```python
from build123d import *

# Parameters (mm, degrees)
SKETCH1_W               = 38.1508
SKETCH1_H               = 9.525
CUT_EXTRUDE1_DEPTH      = 55.787705795
CUT_EXTRUDE1_DEPTH_BACK = 55.787705795
SKETCH2_R               = 11.8745
SKETCH2_R_2             = 3.175
CUT_EXTRUDE2_DEPTH      = 55.787705795
CUT_EXTRUDE2_DEPTH_BACK = 55.787705795
SKETCH3_R               = 3.175
SKETCH4_R               = 2.3749
CUT_EXTRUDE3_DEPTH      = 6.35
CIRPATTERN1_COUNT       = 3


with BuildPart() as part:
    # Sketch1 → Revolve1 (revolve)
    with BuildSketch(Plane.XY, mode=Mode.PRIVATE) as revolve1_sk:
        with Locations((19.0754, 4.7625)):
            Rectangle(SKETCH1_W, SKETCH1_H)
    revolve(revolve1_sk.sketch.rotate(Axis((0, 0, 0), (0, 1, 0)), 90), axis=Axis((0, 0, 0), (0, 1, 0)))

    # Sketch2 → Cut-Extrude1 (cut, two sides: drawn at the far end of the back side and taken through both)
    with BuildSketch(Plane(origin=(0, 9.525, 0), x_dir=(1, 0, 0), z_dir=(0, 1, 0)).offset(-CUT_EXTRUDE1_DEPTH_BACK)):
        with Locations(Location((-12.7, 14.986, 0), (0, 0, 270))):
            Circle(SKETCH2_R)
        with Locations(Location((12.7, 14.986, 0), (0, 0, 270))):
            Circle(SKETCH2_R)
        with Locations(Location((0, 25.146, 0), (0, 0, 270))):
            Circle(SKETCH2_R_2)
        with Locations(Location((0, 4.826, 0), (0, 0, 270))):
            Circle(SKETCH2_R_2)
        with Locations(Location((0, -14.605, 0), (0, 0, 270))):
            Circle(SKETCH2_R_2)
    extrude(amount=CUT_EXTRUDE1_DEPTH + CUT_EXTRUDE1_DEPTH_BACK, mode=Mode.SUBTRACT)

    # Sketch3 → Cut-Extrude2 (cut, two sides: drawn at the far end of the back side and taken through both)
    with BuildSketch(Plane(origin=(0, 9.525, 0), x_dir=(1, 0, 0), z_dir=(0, 1, 0)).offset(-CUT_EXTRUDE2_DEPTH_BACK)):
        with Locations(Location((-25.4, -1.27, 0), (0, 0, 270))):
            Circle(SKETCH3_R)
        with Locations(Location((25.4, -1.27, 0), (0, 0, 270))):
            Circle(SKETCH3_R)
    extrude(amount=CUT_EXTRUDE2_DEPTH + CUT_EXTRUDE2_DEPTH_BACK, mode=Mode.SUBTRACT)

    # Sketch4 → Cut-Extrude3 (cut)
    with BuildSketch(Plane(origin=(33.039561975, 0, 19.0754), x_dir=(0, -1, 0), z_dir=(0.866025403784438, 0, 0.500000000000001))):
        with Locations(Location((-4.7625, 0, 0), (0, 0, 90))):
            Circle(SKETCH4_R)
    cut_extrude3 = extrude(amount=-CUT_EXTRUDE3_DEPTH, mode=Mode.SUBTRACT)

    # CirPattern1: Cut-Extrude3 ×3 about axis
    cirpattern1_axis = Axis((0, 0, 0), (0, 1, 0))
    for i in range(1, CIRPATTERN1_COUNT):
        add(cut_extrude3.rotate(cirpattern1_axis, i * 360 / CIRPATTERN1_COUNT), mode=Mode.SUBTRACT)


solid = part.part
```
Could you check a few things on this model? Use its own coordinates, in mm. A direction names the side the tool comes from. Coordinates: 2 decimals unless noted, no trailing zeros. Order: outer loops, then holes, each group sorted by start corner. A loop starts at its lowest first (then second) coordinate and runs counter-clockwise, first axis right, second up. Notation, with made-up numbers: M 49.5,30.5 L 63.5,30.5 A19 cw 63.5,41.5 Z; hole C 68.25,-25.5 d1. An arc over 180 degrees is marked long. Use a Markdown table: item, result. Add a question column.
Q1. We'd pull the mould along X, two halves only. Please class faces 4 (the flat face through (-1, 9.525, 8)), 5 (the cylindrical face through (0.14, 4.696, 11.433)), 6 (the cylindrical face through (23.21, 4.83, 30.28)): pulls with the +X half, pulls with the -X half, needs draft (parallel to the pull), parting line crosses it, or undercut.
Q2. Which directions (+Z, -Z, +X, -X, +Y, -Y) give clear straight access to the entire face, cutting with the end or side of a thin tool? Please do faces 1 (the flat face through (-1, 0, 8)), 2 (the flat face through (-27.56, 4.8, 15.87)), 3 (the cylindrical face through (1.75, 6.37, -35.02)).
Q3. I want a section at C-C on x = 19. List the corners of the cut face in (y, z) for me (3 decimals), then the cut area to 3 significant figures.
Q4. I want a section at D-D on z = -18.5. List the corners of the cut face in (x, y) for me (3 decimals), then the cut area to 3 significant figures.
Q5. I'm going to push flat-ended pins straight in: pin 1 (2 mm diameter, centred on x = -21.5, y = 5.5, fed in from +Z); pin 2 (4 mm diameter, centred on x = -25.4, z = 1.27, fed in from -Y); pin 3 (2.5 mm diameter, centred on x = 1, y = 4.5, fed in from -Z); pin 4 (3 mm diameter, centred on y = 7.5, z = 7, fed in from +X). Where does each tip first touch, or does it pass through?
Q6. I want a section at B-B on z = 3. List the corners of the cut face in (x, y) for me (3 decimals), then the cut area to 3 significant figures.
Q7. If I drill on L1, parallel to Z at x = 0, y = 4.75; L2, parallel to Y at x = 0, z = -35 (3 decimals); L3, parallel to X at y = 7.75, z = 1.27 (3 decimals), over which ranges is the centre line in solid material (lowest first)?
Q8. I want a section at A-A on x = 9.5. List the corners of the cut face in (y, z) for me (3 decimals).
Checked values:
| question | item | result |
|---|---|---|
| 1 | face 4 | needs draft |
| 1 | face 5 | undercut |
| 1 | face 6 | parting line crosses it |
| 2 | face 1 | +Z, -Z, +X, -X, -Y |
| 2 | face 2 | none |
| 2 | face 3 | -Z |
| 3 | outline | M 0,-33.083 L 9.525,-33.083 L 9.525,-25.051 L 0,-25.051 Z; M 0,-4.921 L 9.525,-4.921 L 9.525,33.083 L 0,33.083 Z |
| 3 | area | 438 mm² |
| 4 | outline | M -33.365,0 L -24.043,0 L -24.043,9.525 L -33.365,9.525 Z; M -1.357,0 L 1.357,0 L 1.357,9.525 L -1.357,9.525 Z; M 24.043,0 L 33.365,0 L 33.365,9.525 L 24.043,9.525 Z |
| 4 | area | 203 mm² |
| 5 | pin 1 | z = 32.18 |
| 5 | pin 2 | through |
| 5 | pin 3 | z = -31.8 |
| 5 | pin 4 | x = 37.75 |
| 6 | outline | M -38.033,0 L -28.062,0 L -28.062,9.525 L -38.033,9.525 Z; M -22.738,0 L 22.738,0 L 22.738,9.525 L -22.738,9.525 Z; M 28.062,0 L 38.033,0 L 38.033,9.525 L 28.062,9.525 Z |
| 6 | area | 623 mm² |
| 7 | L1 | -31.8 to -28.32, -21.97 to -8, -1.65 to 11.43, 17.78 to 38.15 |
| 7 | L2 | 0 to 2.388, 7.137 to 9.525 |
| 7 | L3 | -38.13 to -28.575, -22.225 to 22.225, 28.575 to 38.13 |
| 8 | outline | M 0,-36.949 L 9.525,-36.949 L 9.525,-26.421 L 0,-26.421 Z; M 0,-3.551 L 9.525,-3.551 L 9.525,36.949 L 0,36.949 Z |
